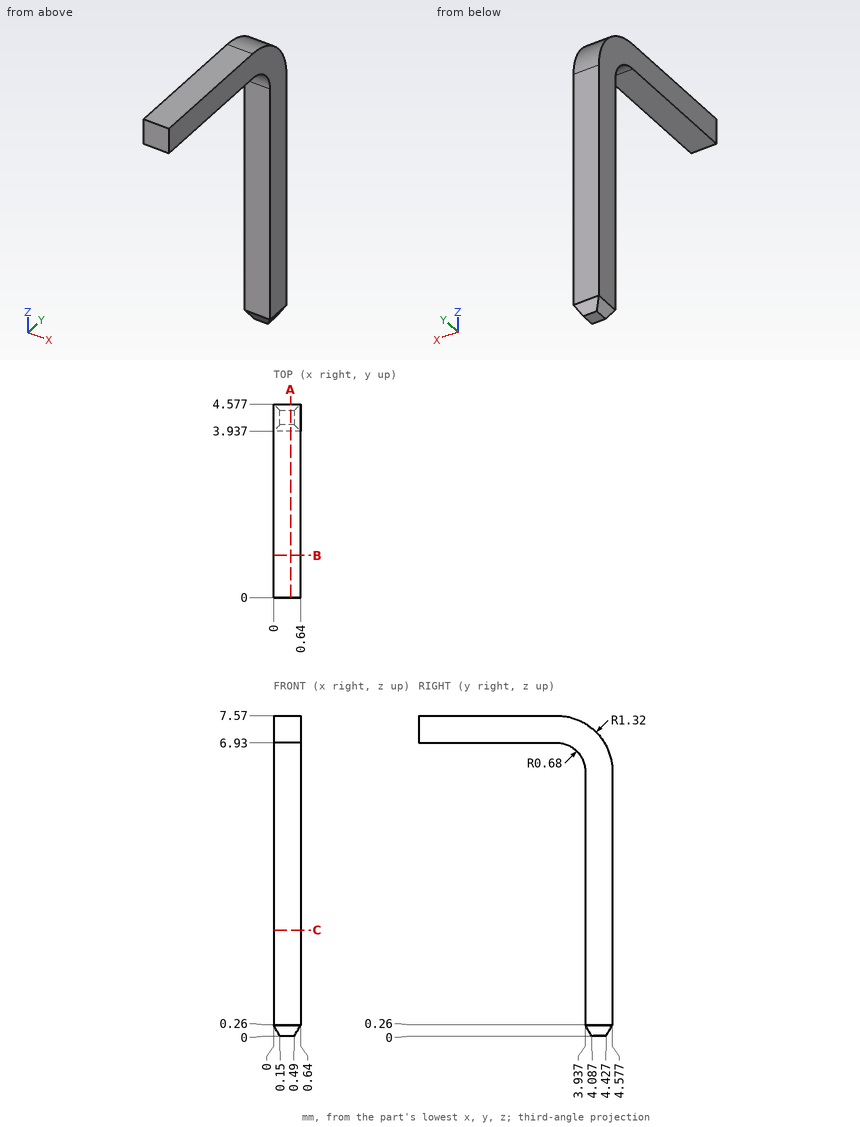
Geometry check sheet. Reference: drawing and pictorial views, mm from the part's lowest x, y, z. Round coordinates to 2 decimals unless told otherwise and drop trailing zeros. Loops run counter-clockwise (first coordinate to the right, second up) from the corner with the lowest first, then second, coordinate; pieces in that order, holes last.
1. Gauge pin test, flat end, axial feed: pin 1 Ø2 at (y, z) = (2, 5) entering from -X. Record the tip position at first contact, or that the pin passes through.
2. Scan lines: probe 1 along Y at (x, z) = (0.55, 1.75); probe 2 along Z at (x, y) = (0.45, 3); probe 3 along Y at (x, z) = (0.05, 6.75). Record each from-to range of solid material in increasing order.
3. Sectioned sample at A-A on x = 0.4. Record the boundary of the cut face in (y, z).
4. Sectioned sample at B-B on y = 1. Record the boundary of the cut face in (x, z).
5. Sectioned sample at C-C on z = 2.5. Record the boundary of the cut face in (x, y).
Recorded:
1. pin 1: passes through
2. probe 1: y = 3.94 to 4.58
2. probe 2: z = 6.93 to 7.57
2. probe 3: y = 3.72 to 4.48
3. outline: (0, 6.93) - (3.26, 6.93) arc R0.68 cw to (3.94, 6.25) - (3.94, 0.26) - (4.09, 0) - (4.43, 0) - (4.58, 0.26) - (4.58, 6.25) arc R1.32 ccw to (3.26, 7.57) - (0, 7.57) - close
4. outline: (0, 6.93) - (0.64, 6.93) - (0.64, 7.57) - (0, 7.57) - close
5. outline: (0, 3.94) - (0.64, 3.94) - (0.64, 4.58) - (0, 4.58) - close
